from build123d import *

# Parameters (mm, degrees)
ESBO_O1_W                = 20
ESBO_O1_H                = 50
ESBO_O1_R                = 2
ESBO_O1_W_2              = 50
ESBO_O1_H_2              = 20
RESSALTO_EXTRUS_O1_DEPTH = 3


with BuildPart() as part:
    # Esboço1 → Ressalto-extrusão1 (new body)
    with BuildSketch(Plane(origin=(0, 0, 0), x_dir=(0, 0, -1), z_dir=(1, 0, 0))):
        with Locations((10, 45)):
            Rectangle(ESBO_O1_W, ESBO_O1_H)
        with Locations((10, 35)):
            Circle(ESBO_O1_R, mode=Mode.SUBTRACT)
        with Locations((10, 55)):
            Circle(ESBO_O1_R, mode=Mode.SUBTRACT)
        with Locations((45, 10)):
            Rectangle(ESBO_O1_W_2, ESBO_O1_H_2)
        with Locations((35, 10)):
            Circle(ESBO_O1_R, mode=Mode.SUBTRACT)
        with Locations((55, 10)):
            Circle(ESBO_O1_R, mode=Mode.SUBTRACT)
        with Locations((10, 10)):
            Rectangle(ESBO_O1_W, ESBO_O1_H_2)
    extrude(amount=RESSALTO_EXTRUS_O1_DEPTH)


solid = part.part
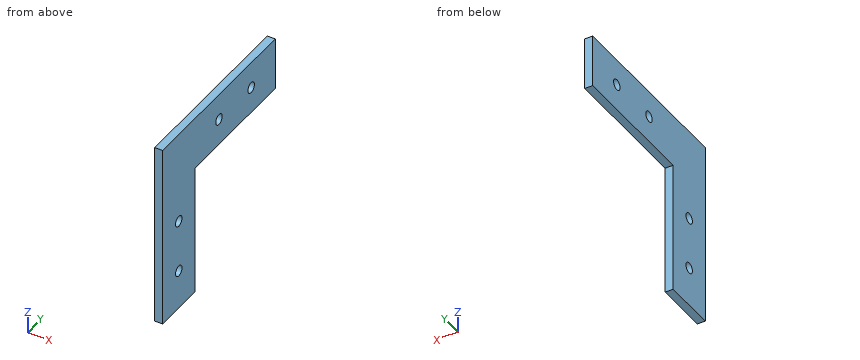
For this review, take the finished solid that the model builds, in its own axes (mm). Coordinates: 2 decimals unless noted, no trailing zeros. Order: outer loops, then holes, each group sorted by start corner. A loop starts at its lowest first (then second) coordinate and runs counter-clockwise, first axis right, second up. Notation, with made-up numbers: (13, 6.25) -> (20, 6.25) arc R25 cw to (20, 31.25) -> close; hole circle Ø9 at (-20.75, -20.5). An arc over 180 degrees is marked (long way). Return JSON: item names as keys, results as strings.
1. We need section C-C on x = 2.5. Write out the cut boundary in (y, z).
Answer block:
{"outline": "(0, -70) -> (20, -70) -> (20, -20) -> (70, -20) -> (70, 0) -> (0, 0) -> close; hole circle Ø4 at (10, -55); hole circle Ø4 at (10, -35); hole circle Ø4 at (35, -10); hole circle Ø4 at (55, -10)"}
2. We need section B-B on z = -55. Write out the cut boundary in (x, y), and give its area (3 significant figures).
Answer block:
{"outline": "(0, 0) -> (3, 0) -> (3, 8) -> (0, 8) -> close; (0, 12) -> (3, 12) -> (3, 20) -> (0, 20) -> close", "area": "48.0 mm²"}
3. We need section D-D on y = 35. Write out the cut boundary in (x, z), and give its area (3 significant figures).
Answer block:
{"outline": "(0, -20) -> (3, -20) -> (3, -12) -> (0, -12) -> close; (0, -8) -> (3, -8) -> (3, 0) -> (0, 0) -> close", "area": "48.0 mm²"}
4. For line 1 (Y direction, x = 0.8, z = -10); line 2 (Y direction, x = 1.75, z = -35); line 3 (Z direction, x = 1.35, y = 36), list the stretches that pass through material, from the lowest coordinate up. Write a range as from..to.
Answer block:
{"line 1": "0..33, 37..53, 57..70", "line 2": "0..8, 12..20", "line 3": "-20..-11.73, -8.27..0"}
5. For pin 1 Ø3.5 at (y, z) = (55, -10) entering from -X; pin 2 Ø1.5 at (x, y) = (1.5, 55) entering from -Z; pin 3 Ø1.5 at (x, z) = (1, -52.5) entering from +Y, all flat-tipped, find the tip position at first contact; note any pin that passes through.
Answer block:
{"pin 1": "through", "pin 2": "z = -20", "pin 3": "y = 20"}
6. We need section A-A on y = 10. Write out the cut boundary in (x, z).
Answer block:
{"outline": "(0, -70) -> (3, -70) -> (3, -57) -> (0, -57) -> close; (0, -53) -> (3, -53) -> (3, -37) -> (0, -37) -> close; (0, -33) -> (3, -33) -> (3, 0) -> (0, 0) -> close"}
